Could you check a few things on this model? Use its own coordinates, in mm. Face numbers are marked on the shaded views. A direction names the side the tool comes from. Give positions to 0.01 mm unless a question says otherwise; leave off trailing zeros. Order: outer loops, then holes, each group sorted by start corner. A loop starts at its lowest first (then second) coordinate and runs counter-clockwise, first axis right, second up. Notation, with made-up numbers: M 80,70 L 127,70 A7 ccw 127,76 Z; hole C 87.25,10.5 d2. An arc over 180 degrees is marked long. Use a Markdown table: item, result. Add a question column.
Item 1: For the marked faces 4, 5 and 6, which set-ups out of +Z, -Z, +X, -X, +Y, -Y let a thin tool reach every point of the face, with its end or its side?
Item 2: If I drill on L1, parallel to X at y = -1.5, z = 17.25; L2, parallel to Z at x = -7, y = 0; L3, parallel to Y at x = -5.7, z = 11.43, over which ranges is the centre line in solid material (lowest first)? Write a range as from..to.
Item 3: Suppose I cut it at B-B on z = 11.43. Write out the boundary of the cut face in (x, y), plus the area to 3 significant figures.
Item 4: If we mould it in two halves opening along Z, with no side actions, what happens to the marked faces 1, 2 and 3? For each: released by +Z, released by -Z, zero draft, split by the parting line, or undercut.
Item 5: Suppose I cut it at C-C on z = 6. Write out the boundary of the cut face in (x, y).
Item 6: I'm going to push flat-ended pins straight in: pin 1 Ø4 at (x, y) = (-18.86, 0) entering from +Z; pin 2 Ø4 at (y, z) = (-1, 8.5) entering from +X; pin 3 Ø3 at (y, z) = (0, 9) entering from +X. Where does each tip first touch, or does it pass through?
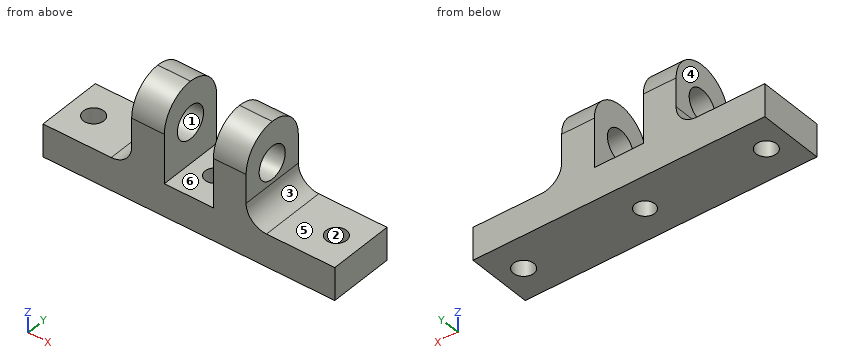
Autodesk Inventor part; units mm, degrees
ref_plane "YZ Plane" through (0, 0, 0) normal (1, 0, 0) x (0, 1, 0)
ref_plane "XZ Plane" through (0, 0, 0) normal (0, 1, 0) x (-1, 0, 0)
ref_plane "XY Plane" through (0, 0, 0) normal (0, 0, 1) x (1, 0, 0)
sketch "Sketch1" plane through (0, 0, 0) normal (0, 0, 1) x (1, 0, 0)
  line L0 (-22.6695, -5.08) -> (22.6695, -5.08)
  line L1 (22.6695, -5.08) -> (22.6695, 5.08)
  line L2 (22.6695, 5.08) -> (-22.6695, 5.08)
  line L3 (-22.6695, 5.08) -> (-22.6695, -5.08)
  line L4 (-22.6695, -5.08) -> (22.6695, 5.08) construction
  line L5 (22.6695, -5.08) -> (-22.6695, 5.08) construction
  point P0 (0, 0)
  dimension "d0" = 10.16
  dimension "d1" = 45.339
extrude "Extrusion1" add sketch "Sketch1" along normal blind 5.08
sketch "Sketch2" plane through (0, 0, 0) normal (0, 0, -1) x (-1, 0, 0)
  line L0 (22.6695, 5.08) -> (22.6695, -5.08)
  line L1 (-22.6695, -5.08) -> (-22.6695, 5.08)
  line L2 (-22.6695, 5.08) -> (22.6695, 5.08)
  point P0 (0, 0)
  point P1 (18.8595, 0)
  point P2 (-18.8595, 0)
  dimension "d4" = 3.81
  dimension "d5" = 3.81
  dimension "d6" = 5.08
  dimension "d7" = 5.08
hole "Hole1" at (-18.8595, 0, 0) at (18.8595, 0, 0) direction (0, 0, 1) diameter 3.175 end through all
sketch "Sketch3" plane through (0, 0, 0) normal (0, 0, -1) x (-1, 0, 0)
  circle A0 centre (0, 0) radius 1.524
  dimension "d15" = 3.048
extrude "Extrusion2" cut sketch "Sketch3" against normal through all
sketch "Sketch4" plane through (0, 0, 5.08) normal (0, 0, 1) x (1, 0, 0)
  line L0 (22.6695, 5.08) -> (-22.6695, 5.08)
  line L1 (-22.6695, -5.08) -> (22.6695, -5.08)
  line L2 (-3.81, 5.08) -> (-8.89, 5.08)
  line L3 (-8.89, 5.08) -> (-8.89, -5.08)
  line L4 (-8.89, -5.08) -> (-3.81, -5.08)
  line L5 (-3.81, -5.08) -> (-3.81, 5.08)
  line L6 (3.81, 5.08) -> (8.89, 5.08)
  line L7 (8.89, 5.08) -> (8.89, -5.08)
  line L8 (8.89, -5.08) -> (3.81, -5.08)
  line L9 (3.81, -5.08) -> (3.81, 5.08)
  point P0 (0, 0)
  dimension "d18" = 5.08
  dimension "d19" = 3.81
  dimension "d20" = 3.81
  dimension "d21" = 5.08
extrude "Extrusion3" add sketch "Sketch4" along normal blind 12.7 contours L7 L1 L9 L0 | L5 L1 L3 L0
sketch "Sketch5" plane through (-8.89, -5.08, 5.08) normal (-1, 0, 0) x (0, 0, 1)
  line L0 (12.7, 10.16) -> (12.7, 0)
  line L1 (0, 10.16) -> (12.7, 10.16)
  point P0 (-5.08, 5.08)
  point P1 (6.35, 5.08)
  dimension "d24" = 6.35
  dimension "d25" = 5.08
hole "Hole2" at (-8.89, 0, 11.43) direction (1, 0, 0) diameter 5.08 end through all
fillet "Fillet1" radius 3.175 2 edges at (-8.89, 0, 5.08) (8.89, 0, 5.08)
fillet "Fillet2" radius 5.08 4 edges at (6.35, -5.08, 17.78) (6.35, 5.08, 17.78) (-6.35, -5.08, 17.78) (-6.35, 5.08, 17.78)
properties part number "LowerSpringMountFront"
Findings below:
| question | item | result |
|---|---|---|
| 1 | face 4 | +Z, -X, +Y, -Y |
| 1 | face 5 | +Z, +X, +Y, -Y |
| 1 | face 6 | +Z, +Y, -Y |
| 2 | L1 | x = -8.89..-3.81, 3.81..8.89 |
| 2 | L2 | z = 0..8.89, 13.97..17.78 |
| 2 | L3 | y = -5.08..-2.54, 2.54..5.08 |
| 3 | outline | M -8.89,-5.08 L -3.81,-5.08 L -3.81,-2.54 L -8.89,-2.54 Z; M -8.89,2.54 L -3.81,2.54 L -3.81,5.08 L -8.89,5.08 Z; M 3.81,-5.08 L 8.89,-5.08 L 8.89,-2.54 L 3.81,-2.54 Z; M 3.81,2.54 L 8.89,2.54 L 8.89,5.08 L 3.81,5.08 Z |
| 3 | area | 51.6 mm^2 |
| 4 | face 1 | undercut |
| 4 | face 2 | zero draft |
| 4 | face 3 | released by +Z |
| 5 | outline | M -9.83,-5.08 L -3.81,-5.08 L -3.81,5.08 L -9.83,5.08 Z; M 3.81,-5.08 L 9.83,-5.08 L 9.83,5.08 L 3.81,5.08 Z |
| 6 | pin 1 | stops at z = 5.08 |
| 6 | pin 2 | stops at x = 9.42 |
| 6 | pin 3 | stops at x = 8.98 |
